Source: CAD feature listing. Evaluate the final solid. Frame: model axes, mm. A direction names the side the tool comes from. Coordinates: 2 decimals unless noted, no trailing zeros. Order: outer loops, then holes, each group sorted by start corner. A loop starts at its lowest first (then second) coordinate and runs counter-clockwise, first axis right, second up.
```python
from build123d import *

# Parameters (mm, degrees)
BOSS_EXTRUDE1_START         = -11.086796564
BOSS_EXTRUDE1_OUTLINE_W     = 199.999998902
BOSS_EXTRUDE1_OUTLINE_H     = 6.35
BOSS_EXTRUDE1_DEPTH         = 11.596668503
BOSS_EXTRUDE1_START_2       = -17.436796564
BOSS_EXTRUDE1_2_OUTLINE_W   = 10
BOSS_EXTRUDE1_2_OUTLINE_H   = 6.35
BOSS_EXTRUDE1_2_OUTLINE_W_2 = 9.999999878
BOSS_EXTRUDE1_2_DEPTH       = 22.436796492
BOSS_EXTRUDE1_3_OUTLINE_W   = 16.35
BOSS_EXTRUDE1_3_OUTLINE_H   = 6.35
BOSS_EXTRUDE1_3_DEPTH       = 4.999999928
SKETCH2_W                   = 199.999998902
SKETCH2_H                   = 3.175
CUT_EXTRUDE1_DEPTH          = 3.175


# Read off the part's stored shape, not the designer's step: Boss-Extrude1
with BuildPart() as part:
    # Boss-Extrude1 outline → Boss-Extrude1 (new body)
    with BuildSketch(Plane(origin=(0, 0, 0), x_dir=(1, 0, 0), z_dir=(0, 1, 0)).offset(BOSS_EXTRUDE1_START)):
        with Locations((106.349999451, -3.175)):
            Rectangle(BOSS_EXTRUDE1_OUTLINE_W, BOSS_EXTRUDE1_OUTLINE_H)
    extrude(amount=BOSS_EXTRUDE1_DEPTH)



with BuildPart() as body_2:
    # Boss-Extrude1 2 outline → Boss-Extrude1 2 (new body)
    with BuildSketch(Plane(origin=(0, 0, 0), x_dir=(1, 0, 0), z_dir=(0, 1, 0)).offset(BOSS_EXTRUDE1_START_2)):
        Polygon((76.349999756, 0), (76.349999756, -6.35), (86.349999688, -6.35), (86.349999634, 0), align=None)
        Polygon((56.349999878, -6.35), (66.349999811, -6.35), (66.349999865, 0), (56.349999878, 0), align=None)
        Polygon((96.349999634, 0), (96.349999634, -6.35), (106.349999567, -6.35), (106.349999512, 0), align=None)
        Polygon((36.35, -6.35), (46.349999932, -6.35), (46.349999987, 0), (36.35, 0), align=None)
        Polygon((116.349999512, 0), (116.349999512, -6.35), (126.349999444, -6.35), (126.34999939, 0), align=None)
        with Locations((21.35, -3.175)):
            Rectangle(BOSS_EXTRUDE1_2_OUTLINE_W, BOSS_EXTRUDE1_2_OUTLINE_H)
        Polygon((136.34999939, 0), (136.34999939, -6.35), (146.349999322, -6.35), (146.349999268, 0), align=None)
        Polygon((156.349999268, 0), (156.349999268, -6.35), (166.349999201, -6.35), (166.349999146, 0), align=None)
        Polygon((176.349999146, 0), (176.349999146, -6.35), (186.349999078, -6.35), (186.349999024, 0), align=None)
        with Locations((201.349998963, -3.175)):
            Rectangle(BOSS_EXTRUDE1_2_OUTLINE_W_2, BOSS_EXTRUDE1_2_OUTLINE_H)
    extrude(amount=BOSS_EXTRUDE1_2_DEPTH)


with BuildPart() as part_1:
    add(part.part)

    add(body_2.part)  # Boss-Extrude1 3 merges body 2
    # Boss-Extrude1 3 outline → Boss-Extrude1 3 (add)
    with BuildSketch(Plane(origin=(0, 0, 0), x_dir=(1, 0, 0), z_dir=(0, 1, 0))):
        with Locations((8.175, -3.175)):
            Rectangle(BOSS_EXTRUDE1_3_OUTLINE_W, BOSS_EXTRUDE1_3_OUTLINE_H)
        Polygon((206.349998902, 0), (206.349998902, -6.35), (212.699998902, -6.35), (212.699998619, 0), align=None)
    extrude(amount=BOSS_EXTRUDE1_3_DEPTH)

    # Sketch2 → Cut-Extrude1 (cut)
    with BuildSketch(Plane.XY.offset(6.35)):
        with Locations((106.349999451, -4.252628114)):
            Rectangle(SKETCH2_W, SKETCH2_H)
    extrude(amount=-CUT_EXTRUDE1_DEPTH, mode=Mode.SUBTRACT)


solid = part_1.part
```
1. Pin query (flat end, axial travel): P1, Ø1.9, axis at y = -15.5, z = 2.5, coming from the +X side; P2, Ø3.5, axis at x = 75.5, y = -3.5, coming from the +Z side; P3, Ø1.5, axis at x = 112.5, z = 2, coming from the +Y side; P4, Ø1.9, axis at y = -4.5, z = 4, coming from the -X side. Return the tip coordinate at first contact, or that it passes through.
Findings:
P1: stops at x = 206.35
P2: stops at z = 6.35
P3: stops at y = 0.51
P4: stops at x = 6.35
2. Section query A-A on x = 130.5. Return loops of the section in (y, z) (3 decimals).
Findings:
outline: (-11.087, 0) - (0.51, 0) - (0.51, 6.35) - (-2.665, 6.35) - (-2.665, 3.175) - (-5.84, 3.175) - (-5.84, 6.35) - (-11.087, 6.35) - close
3. Ray query, line 1 (Y direction, x = 40, z = 3.75); line 2 (Y direction, x = 9.5, z = 5); line 3 (Y direction, x = 9.5, z = 2.5). Return the intervals inside material, ascending.
Findings:
line 1: y = -17.44 to -5.84, -2.67 to 5
line 2: y = -11.09 to -5.84, -2.67 to 5
line 3: y = -11.09 to 5
4. Section query C-C on x = 40.5. Return loops of the section in (y, z) (3 decimals).
Findings:
outline: (-17.437, 0) - (5, 0) - (5, 6.35) - (-2.665, 6.35) - (-2.665, 3.175) - (-5.84, 3.175) - (-5.84, 6.35) - (-17.437, 6.35) - close
5. Draft query along X for faces 4 (the face through (156.35, 3, 3)), 5 (the face through (21, -17.437, 3)). Return one class per face: released by +X, released by -X, zero draft, split by the parting line, or undercut.
Findings:
face 4: undercut
face 5: zero draft
6. Access query for faces 1 (the face through (56.35, 3, 3)), 2 (the face through (111, -11.087, 3)), 3 (the face through (81, 5, 3)). Directions: +Z, -Z, +X, -X, +Y, -Y. A direction counts if a zero-diameter tool reaches every point of the face in a straight line with its end or side. Return the directions, or none.
Findings:
face 1: +Z, -Z, +Y
face 2: +Z, -Z, -Y
face 3: +Z, -Z, +X, -X, +Y
7. Section query B-B on y = -8. Return loops of the section in (x, z).
Findings:
outline: (6.35, 0) - (206.35, 0) - (206.35, 6.35) - (6.35, 6.35) - close
